Verification items for the finished model (mm, model axes). A direction names the side the tool comes from. Round coordinates to 2 decimals unless told otherwise and drop trailing zeros. Order: outer loops, then holes, each group sorted by start corner. A loop starts at its lowest first (then second) coordinate and runs counter-clockwise, first axis right, second up. Notation, with made-up numbers: M -2.75,66 L 52.25,66 A23 ccw 52.25,86 Z; hole C -15,62 d3. An arc over 180 degrees is marked long. Write item = value, one per line. Start each with the question number.
from build123d import *

# Parameters (mm, degrees)
BASE_EXTRUDE_DEPTH       = 10
BOSS_EXTRUDE1_DEPTH      = 8
SKETCH3_R                = 32
BOSS_EXTRUDE2_DEPTH      = 64
SKETCH7_R                = 21
CUT_EXTRUDE1_DEPTH       = 237.258333186
BOSS_EXTRUDE3_REACH      = 233.901
BOSS_EXTRUDE3_END_RADIUS = 32
SKETCH4_W                = 8
SKETCH4_H                = 42
HOLE1_D                  = 20
LPATTERN1_COUNT          = 2
LPATTERN1_PITCH          = 65


with BuildPart() as part:
    # Sketch1 → Base-Extrude (new body)
    with BuildSketch(Plane(origin=(0, 0, 0), x_dir=(1, 0, 0), z_dir=(0, 1, 0))):
        with BuildLine():
            Line((25, 0), (135, 0))
            ThreePointArc((135, 0), (152.67766953, 7.32233047), (160, 25))
            Line((160, 25), (160, 89))
            Line((160, 89), (0, 89))
            Line((0, 89), (0, 25))
            ThreePointArc((0, 25), (7.32233047, 7.32233047), (25, 0))
        make_face()
    extrude(amount=BASE_EXTRUDE_DEPTH)

    # Sketch2 → Boss-Extrude1 (add)
    with BuildSketch(Plane(origin=(0, 0, -89), x_dir=(-1, 0, 0), z_dir=(0, 0, -1))):
        with BuildLine():
            Line((-160, 10), (0, 10))
            ThreePointArc((0, 10), (-1.526648698, 15.857381028), (-5.718152085, 20.224401536))
            Line((-5.718152085, 20.224401536), (-139.248405559, 102.265070762))
            ThreePointArc((-139.248405559, 102.265070762), (-186.188017348, 85.615253581), (-160, 43.250984267))
            Line((-160, 43.250984267), (-160, 10))
        make_face()
    extrude(amount=-BOSS_EXTRUDE1_DEPTH)

    # Sketch3 → Boss-Extrude2 (add)
    with BuildSketch(Plane(origin=(0, 0, -95), x_dir=(-1, 0, 0), z_dir=(0, 0, -1))):
        with Locations((-156, 75)):
            Circle(SKETCH3_R)
    extrude(amount=-BOSS_EXTRUDE2_DEPTH)

    # Sketch7 → Cut-Extrude1 (cut, through all)
    with BuildSketch(Plane(origin=(0, 0, -95), x_dir=(-1, 0, 0), z_dir=(0, 0, -1))):
        with Locations((-156, 75)):
            Circle(SKETCH7_R)
    extrude(amount=-CUT_EXTRUDE1_DEPTH, mode=Mode.SUBTRACT)

    # Boss-Extrude3: up to this cylinder (the profile starts outside it)
    boss_extrude3_end = Plane(origin=(156, 75, -60), z_dir=(0, 0, -1)) * Cylinder(BOSS_EXTRUDE3_END_RADIUS, 532.802, mode=Mode.PRIVATE)
    # Sketch4 → Boss-Extrude3 (add, up to the surface)
    with BuildSketch(Plane(origin=(0, 10, 0), x_dir=(-1, 0, 0), z_dir=(0, 1, 0)), mode=Mode.PRIVATE) as boss_extrude3_sk1:
        with Locations((-156, -60)):
            Rectangle(SKETCH4_W, SKETCH4_H)
    boss_extrude3_tool1 = extrude(boss_extrude3_sk1.sketch, amount=BOSS_EXTRUDE3_REACH, mode=Mode.PRIVATE) - boss_extrude3_end
    add(boss_extrude3_tool1.solids().sort_by_distance((156, 10, -60))[0])

    # Hole1 (through all)
    with Locations(Plane(origin=(0, 10, 0), x_dir=(-1, 0, 0), z_dir=(0, 1, 0))):
        with Locations((-38, -39)):
            hole1 = Hole(HOLE1_D / 2)

    # LPattern1: Hole1 ×2
    with Locations(*[(i * LPATTERN1_PITCH, 0, 0) for i in range(1, LPATTERN1_COUNT)]):
        add(hole1, mode=Mode.SUBTRACT)


solid = part.part
1) Gauge pin test, flat ends, axial feed: P1, Ø4, axis at x = 157.5, y = 32, coming from the +Z side; P2, Ø3, axis at y = 35, z = -42, coming from the -X side; P3, Ø8, axis at y = 65, z = -62, coming from the -X side. Record the tip position at first contact, or that the pin passes through.
2) Scan lines: probe 1 along Y at (x, z) = (156, -56); probe 2 along Z at (x, y) = (103, 5); probe 3 along Y at (x, z) = (149, -33). Record each from-to range of solid material in increasing order.
3) Cross-section at D-D, the plane x = 163.5. Enter the section's corners in (y, z), then the cut area to 3 significant figures.
4) Cross-section at A-A, the plane y = 75. Enter the section's corners in (x, z).
5) Release check for a two-part mould opening along X. For faces 1 (the flat face through (94, 36, -81)), 2 (the flat face through (0, 5, -57)), 3 (the cylindrical face through (100.83, 4.93, -48.76)), 4 (the cylindrical face through (172.665, 62.222, -63.448)) record: pulls with the +X half, pulls with the -X half, needs draft (parallel to the pull), parting line crosses it, or undercut.
6) Cross-section at B-B, the plane z = -75. Enter the section's corners in (x, y), then the cut area to 3 significant figures.
7) Access from +Z, -Z, +X, -X, +Y, -Y to the whole of each face (thin tool, end or side, straight path). Record for faces 5 (the flat face through (160, 21, -65)), 6 (the flat face through (149, 54, -31)), 7 (the flat face through (156, 26, -39)), 8 (the flat face through (152, 26, -60)).
8) Cross-section at C-C, the plane x = 37. Enter the section's corners in (y, z).
Geometry results:
q1.P1 = -39
q1.P2 = 152
q1.P3 = 124.57
q2.probe_1 = 0 to 54, 96 to 107
q2.probe_2 = -89 to -49, -29 to 0
q2.probe_3 = 0 to 10, 43.78 to 55.2, 94.8 to 106.22
q3.outline = M 43.89,-95 L 55.38,-95 L 55.38,-31 L 43.89,-31 Z; M 94.62,-95 L 106.11,-95 L 106.11,-31 L 94.62,-31 Z
q3.area = 1,470 mm^2
q4.outline = M 94.87,-89 L 124,-89 L 124,-95 L 135,-95 L 135,-31 L 124,-31 L 124,-81 L 94.87,-81 Z; M 177,-95 L 188,-95 L 188,-31 L 177,-31 Z
q5.face_1 = needs draft
q5.face_2 = pulls with the -X half
q5.face_3 = undercut
q5.face_4 = undercut
q6.outline = M 0,0 L 160,0 L 160,43.25 A32 ccw long 152,43.25 L 152,10 L 0,10 Z; hole C 156,75 d42
q6.area = 3,700 mm^2
q7.face_5 = +Z, -Z, +X, -Y
q7.face_6 = +Z, +X, -X, +Y
q7.face_7 = +Z, +X, -X
q7.face_8 = +Z, -X
q8.outline = M 0,-89 L 39.44,-89 L 39.44,-81 L 10,-81 L 10,-48.95 L 0,-48.95 Z; M 0,-29.05 L 10,-29.05 L 10,0 L 0,0 Z
